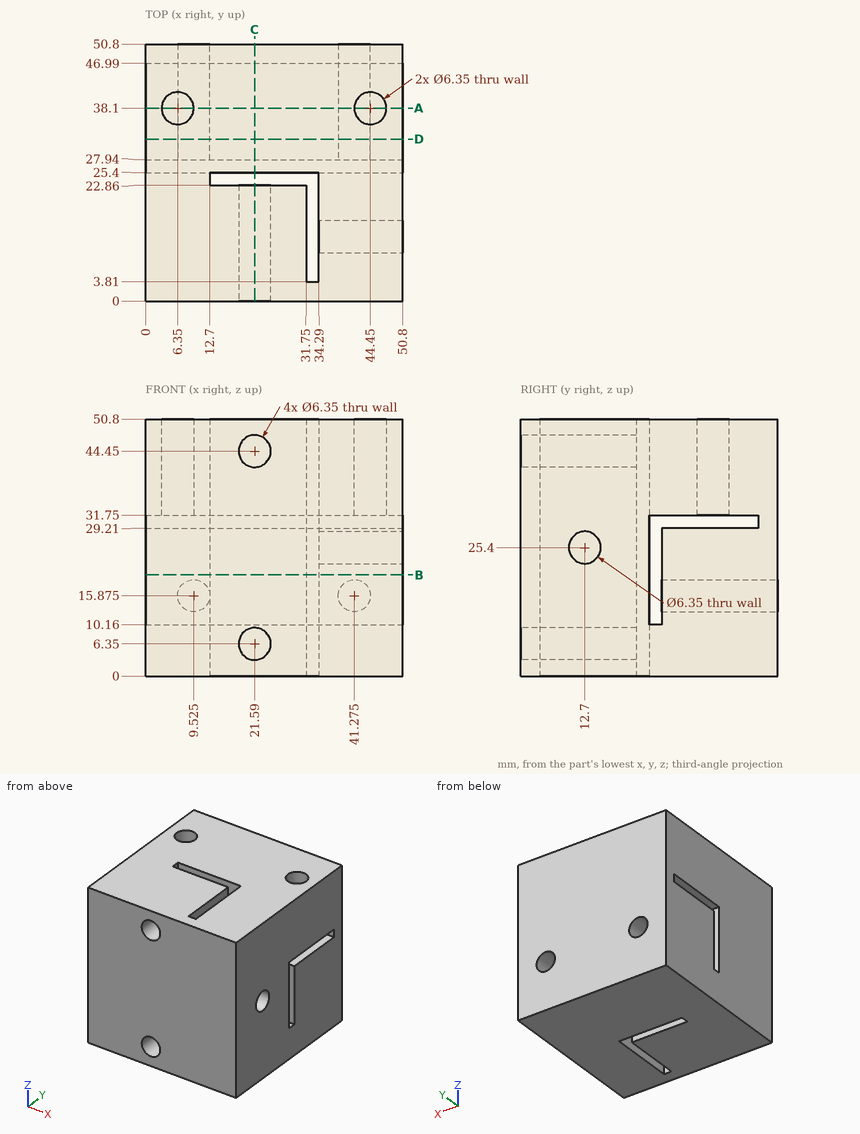
Here's the drawing with two shaded views (mm, measured from the low corner). I have some questions. Coordinates: 2 decimals unless noted, no trailing zeros. Write each loop counter-clockwise with the first axis right and the second up, starting at its lowest first coordinate (ties: lowest second). Pieces come first, ordered by that corner, then holes.
Item 1: I want a section at B-B on z = 20. Write out the boundary of the cut face in (x, y), and give its area (3 significant figures).
Item 2: Will this pin go through, and if not, where does the flat tip stop? pin 1 (4 mm diameter, centred on y = 12.7, z = 25.4, fed in from +X).
Item 3: If I drill on line 1 (Z direction, x = 21.59, y = 6.25) (3 decimals); line 2 (Y direction, x = 6, z = 23.5); line 3 (Z direction, x = 20.5, y = 34), over which ranges is the centre line in solid material (lowest first)?
Item 4: I want a section at A-A on y = 38.1. Write out the boundary of the cut face in (x, z) (3 decimals), and give its area (3 significant figures).
Item 5: I want a section at C-C on x = 21.59. Write out the boundary of the cut face in (y, z) (3 decimals), and give its area (3 significant figures).
Item 6: I want a section at D-D on y = 32. Write out the boundary of the cut face in (x, z) (3 decimals), and give its area (3 significant figures).
Findings below:
1. outline: (0, 0) - (50.8, 0) - (50.8, 25.4) - (34.29, 25.4) - (34.29, 3.81) - (31.75, 3.81) - (31.75, 22.86) - (12.7, 22.86) - (12.7, 25.4) - (0, 25.4) - close; (0, 27.94) - (50.8, 27.94) - (50.8, 50.8) - (0, 50.8) - close
1. area: 2,350 mm2
2. pin 1: stops at x = 31.75
3. line 1: z = 0 to 3.175, 9.525 to 41.275, 47.625 to 50.8
3. line 2: y = 0 to 25.4, 27.94 to 50.8
3. line 3: z = 0 to 29.21, 31.75 to 50.8
4. outline: (0, 0) - (50.8, 0) - (50.8, 29.21) - (0, 29.21) - close; (0, 31.75) - (3.175, 31.75) - (3.175, 50.8) - (0, 50.8) - close; (9.525, 31.75) - (41.275, 31.75) - (41.275, 50.8) - (9.525, 50.8) - close; (47.625, 31.75) - (50.8, 31.75) - (50.8, 50.8) - (47.625, 50.8) - close; hole circle Ø6.35 at (9.525, 15.875); hole circle Ø6.35 at (41.275, 15.875)
4. area: 2,150 mm2
5. outline: (0, 0) - (22.86, 0) - (22.86, 3.175) - (0, 3.175) - close; (0, 9.525) - (22.86, 9.525) - (22.86, 41.275) - (0, 41.275) - close; (0, 47.625) - (22.86, 47.625) - (22.86, 50.8) - (0, 50.8) - close; (25.4, 0) - (50.8, 0) - (50.8, 50.8) - (25.4, 50.8) - (25.4, 31.75) - (46.99, 31.75) - (46.99, 29.21) - (27.94, 29.21) - (27.94, 10.16) - (25.4, 10.16) - close
5. area: 2,060 mm2
6. outline: (0, 0) - (50.8, 0) - (50.8, 29.21) - (0, 29.21) - close; (0, 31.75) - (50.8, 31.75) - (50.8, 50.8) - (0, 50.8) - close; hole circle Ø6.35 at (9.525, 15.875); hole circle Ø6.35 at (41.275, 15.875)
6. area: 2,390 mm2
